The listing builds one solid part. Answer for the finished solid, in the listing's coordinates (mm). Give positions to 0.01 mm unless a question says otherwise; leave off trailing zeros. One line per item, written item: value. Start each with the question number.
Q1. Flat-ended cylindrical pins translate along their axes: pin 1 (10 mm diameter, centred on x = -7, z = 395.5, fed in from +Y); pin 2 (3 mm diameter, centred on y = 0, z = 175.5, fed in from +X); pin 3 (3 mm diameter, centred on x = 4.5, z = -242.5, fed in from +Y); pin 4 (2 mm diameter, centred on x = -6.5, y = 4, fed in from -Z). Find the tip coordinate at first contact, or state that the pin passes through.
Q2. A cutting plane is placed at A-A, the plane z = -371. State how many separate pieces and enclosed holes the cut face has, and give its area (3 significant figures).
Q3. Consider L1, parallel to Y at x = 0, z = 140; L2, parallel to X at y = -7, z = -54; L3, parallel to Y at x = -1.5, z = -237.5. Determine where each line is inside the solid, lowest interval first.
Q4. The mould has two halves that part along Z. Classify faces 1 (the flat face through (1, -3, 500)), 2 (the cylindrical face through (-4.58, 4.29, -7)), 3 (the flat face through (1, -3, -500)): +Z half, -Z half, draft (parallel to the pull), parting line (faces both ways), or undercut.
Autodesk Inventor part; units mm, degrees
ref_plane "YZ Plane" through (0, 0, 0) normal (1, 0, 0) x (0, 1, 0)
ref_plane "XZ Plane" through (0, 0, 0) normal (0, 1, 0) x (-1, 0, 0)
ref_plane "XY Plane" through (0, 0, 0) normal (0, 0, 1) x (1, 0, 0)
sketch "Esboço1" plane through (0, 0, 0) normal (0, 0, 1) x (1, 0, 0)
  line L0 (-10, 10) -> (10, 10) construction
  line L1 (10, 10) -> (10, -10) construction
  line L2 (10, -10) -> (-10, -10) construction
  line L3 (-10, -10) -> (-10, 10) construction
  line L4 (-10, 10) -> (10, -10) construction
  line L5 (10, 10) -> (-10, -10) construction
  circle A0 centre (0, 0) radius 2.5
  line L6 (10, 10) -> (1.7678, 1.7678) construction
  line L7 (1.7678, -1.7678) -> (10, -10) construction
  line L8 (-1.7678, -1.7678) -> (-10, -10) construction
  line L9 (-10, 10) -> (-1.7678, 1.7678) construction
  line L10 (4, 3.1) -> (4, -3.1) construction
  line L11 (-3.1, -5.0193) -> (3.1, -5.0193) construction
  line L12 (3.1, -5.0193) -> (10, -5.0193) construction
  line L13 (-3.1, -5.0193) -> (-10, -5.0193) construction
  line L14 (3.6312, 10) -> (10, 10) construction
  line L15 (3.6312, 10) -> (10, 10) construction
  line L16 (4, 3.1) -> (4, -3.1)
  line L17 (10, 9) -> (10, 4.1)
  line L18 (10, 4.1) -> (9, 4.1)
  line L19 (9, 4.1) -> (9, 3.1)
  line L20 (9, 3.1) -> (8, 3.1)
  line L21 (8, 3.1) -> (8, 6.1)
  arc A1 (8, 6.1) -> (7.275, 6.4381) centre (7.5586, 6.1) ccw
  line L22 (7.275, 6.4381) -> (4.0446, 3.2078)
  arc A2 (4.0446, 3.2078) -> (4, 3.1) centre (4.1524, 3.1) ccw
  line L23 (10, -9) -> (10, -4.1)
  line L24 (10, -4.1) -> (9, -4.1)
  line L25 (9, -4.1) -> (9, -3.1)
  line L26 (9, -3.1) -> (8, -3.1)
  line L27 (8, -3.1) -> (8, -6.1)
  arc A3 (7.275, -6.4381) -> (8, -6.1) centre (7.5586, -6.1) ccw
  arc A4 (4, -3.1) -> (4.0446, -3.2078) centre (4.1524, -3.1) ccw
  line L28 (7.275, -6.4381) -> (4.0446, -3.2078)
  arc A5 (9, -10) -> (10, -9) centre (9, -9) ccw
  arc A6 (10, 9) -> (9, 10) centre (9, 9) ccw
  line L29 (9, -10) -> (4.1, -10)
  line L30 (4.1, -10) -> (4.1, -9)
  line L31 (4.1, -9) -> (3.0767, -9)
  line L32 (3.0767, -9) -> (3.0767, -8)
  line L33 (3.0767, -8) -> (6.0767, -8)
  arc A7 (6.0767, -8) -> (6.4148, -7.275) centre (6.0767, -7.5586) ccw
  line L34 (-3.1233, -4) -> (3.0767, -4)
  arc A8 (3.1845, -4.0446) -> (3.0767, -4) centre (3.0767, -4.1524) ccw
  line L35 (3.1845, -4.0446) -> (6.4148, -7.275)
  arc A9 (-3.1233, -4) -> (-3.1913, -4.0281) centre (-3.1233, -4.0961) ccw
  line L36 (-9, -10) -> (-4.1, -10)
  line L37 (-4.1, -10) -> (-4.1, -9)
  line L38 (-4.1, -9) -> (-3.1, -9)
  line L39 (-3.1, -9) -> (-3.1, -8)
  line L40 (-3.1, -8) -> (-6.1, -8)
  arc A10 (-6.4381, -7.275) -> (-6.1, -8) centre (-6.1, -7.5586) ccw
  line L41 (-3.1913, -4.0281) -> (-6.4381, -7.275)
  arc A11 (-10, -9) -> (-9, -10) centre (-9, -9) ccw
  arc A12 (9, 10) -> (-10, -9) centre (9, -9) ccw
  line L42 (-3.7574, -3.2078) -> (-7.8245, -7.275)
  arc A13 (-3.7574, -3.2078) -> (-3.7127, -3.1) centre (-3.8651, -3.1) ccw
  line L43 (-3.7127, -3.1) -> (-3.7127, 3.1)
  line L44 (7.5486, 8.3855) -> (3.2062, 4.0431)
  arc A14 (-4.1418, 3.3001) -> (-8.8702, -6.8418) centre (9, -9) ccw
  arc A15 (-8.8702, -6.8418) -> (-7.8245, -7.275) centre (-8.2576, -6.8418) ccw
  arc A16 (-3.7127, 3.1) -> (-4.1418, 3.3001) centre (-3.9739, 3.1) ccw
  line L45 (3.0767, 4) -> (-3.1233, 4)
  arc A17 (3.0767, 4) -> (3.2062, 4.0431) centre (3.0984, 4.1509) ccw
  arc A18 (-3.3355, 4.5121) -> (-3.1233, 4) centre (-3.1233, 4.3) ccw
  arc A19 (7.1087, 9.1979) -> (-3.3355, 4.5121) centre (9, -9) ccw
  arc A20 (7.5486, 8.3855) -> (7.1087, 9.1979) centre (7.1604, 8.7006) ccw
  point P0 (4, 0)
  point P1 (4, 0)
  point P2 (8.5, 3.1)
  point P3 (7.7452, 6.5)
  point P4 (7.7452, -6.5)
  point P5 (9.7071, -9.7071)
  point P6 (9.7071, 9.7071)
  point P7 (-6.55, -10)
  point P8 (6.55, -10)
  point P9 (-4.435, 4.435)
  point P10 (-3.7127, 0)
  point P11 (-8.492, -7.4077)
  point P12 (-3.8635, 3.3367)
  point P13 (-0.0233, 4)
  point P14 (-0.0233, -4)
  point P15 (-3.4005, 4.1852)
  point P16 (7.6001, 8.9387)
  dimension "d0" = 20
  dimension "d1" = 20
  dimension "d3" = 5
  dimension "d34" = 1
  dimension "d35" = 1
  dimension "d36" = 2
  dimension "d37" = 130
  dimension "d38" = 6
  dimension "d39" = 6.9
  dimension "d41" = 4.9
  dimension "d42" = 4.9
  dimension "d47" = 45
  dimension "d49" = 3
  dimension "d51" = 13
  dimension "d52" = 4.9
  dimension "d56" = 90
  dimension "d57" = 1
  dimension "d58" = 3
  dimension "d59" = 130
  dimension "d62" = 45
  dimension "d63" = 1.2
  dimension "d64" = 45
  dimension "d65" = 4.9
  dimension "d66" = 1
  dimension "d67" = 1
  dimension "d68" = 1
  dimension "d70" = 3
  dimension "d71" = 130
  dimension "d73" = 90
  dimension "d74" = 19
  dimension "d75" = 6.2
  dimension "d80" = 45
  dimension "d94" = 18
  dimension "d96" = 135
  dimension "d98" = 130
  dimension "d99" = 10.7445
  dimension "d101" = 8
  dimension "d104" = 135
  dimension "d110" = 135
  dimension "d114" = 0.3
extrude "Extrusão1" add sketch "Esboço1" along normal mid plane 1000
properties part number "Ext_003" material "Aço galvanizado"
Answer block:
1. pin 1: y = 6.49
1. pin 2: x = 4
1. pin 3: y = 9.76
1. pin 4: through
2. separate pieces: 1
2. enclosed holes: 3
2. area: 133 mm^2
3. L1: -4 to -2.5, 2.5 to 4, 6.93 to 7.73
3. L2: -9.89 to -8.85, -7.55 to -6.16, 6.14 to 10
3. L3: -4 to -2, 2 to 4, 5.98 to 6.84
4. face 1: +Z half
4. face 2: draft
4. face 3: -Z half
